Verification items for the finished model (mm, model axes). A direction names the side the tool comes from. Give positions to 0.01 mm unless a question says otherwise; leave off trailing zeros. Loops run counter-clockwise (first coordinate to the right, second up) from the corner with the lowest first, then second, coordinate; pieces in that order, holes last. Notation, with made-up numbers: (-5, 14.5) -> (17, 14.5) arc R22 cw to (17, 25.5) -> close; hole circle Ø7 at (37.5, 76). An arc over 180 degrees is marked (long way). Use one line per item in the form item = value. Start each with the question number.
from build123d import *

# Parameters (mm, degrees)
SKETCH1_R           = 5.75
SKETCH1_R_2         = 2
BOSS_EXTRUDE1_DEPTH = 10


with BuildPart() as part:
    # Sketch1 → Boss-Extrude1 (new body)
    with BuildSketch(Plane(origin=(0, 0, 0), x_dir=(1, 0, 0), z_dir=(0, 1, 0))):
        with BuildLine():
            Line((-216.382104852, 37.479356926), (33.317969978, 39.953751753))
            ThreePointArc((33.317969978, 39.953751753), (63.615239274, 9.952328714), (33.312178481, -20.043244588))
            Line((33.312178481, -20.043244588), (-216.38741399, -17.520642817))
            Line((-216.38741399, -17.520642817), (-216.382104852, 37.479356926))
        make_face()
        with Locations((33.615239414, 9.955224607)):
            Circle(SKETCH1_R, mode=Mode.SUBTRACT)
        with Locations((53.615239414, 9.955224607)):
            Circle(SKETCH1_R_2, mode=Mode.SUBTRACT)
        with Locations((43.615239414, -7.365283468)):
            Circle(SKETCH1_R_2, mode=Mode.SUBTRACT)
        with Locations((23.615239414, -7.365283468)):
            Circle(SKETCH1_R_2, mode=Mode.SUBTRACT)
        with Locations((13.615239414, 9.955224607)):
            Circle(SKETCH1_R_2, mode=Mode.SUBTRACT)
        with Locations((23.615239414, 27.275732683)):
            Circle(SKETCH1_R_2, mode=Mode.SUBTRACT)
        with Locations((43.615239414, 27.275732683)):
            Circle(SKETCH1_R_2, mode=Mode.SUBTRACT)
        with BuildLine():
            Line((-176.512574007, 22.873706291), (-121.518027204, 23.418672976))
            ThreePointArc((-121.518027204, 23.418672976), (-107.935613387, 9.968888481), (-121.52062356, -3.478273548))
            Line((-121.52062356, -3.478273548), (-176.515064128, -2.922689649))
            ThreePointArc((-176.515064128, -2.922689649), (-189.283603246, 9.976740986), (-176.512574007, 22.873706291))
        make_face(mode=Mode.SUBTRACT)
        with BuildLine():
            Line((-81.524666784, -3.882334565), (-26.530226217, -4.437918464))
            ThreePointArc((-26.530226217, -4.437918464), (-11.985090745, 9.959626398), (-26.527446362, 24.359979069))
            Line((-26.527446362, 24.359979069), (-81.521993165, 23.815012384))
            ThreePointArc((-81.521993165, 23.815012384), (-95.234126773, 9.967662409), (-81.524666784, -3.882334565))
        make_face(mode=Mode.SUBTRACT)
    extrude(amount=BOSS_EXTRUDE1_DEPTH)


solid = part.part
Item 1: Sectioned sample at D-D, the plane z = -1.5. Enter the section's corners in (x, y), and give its area (3 significant figures).
Item 2: Tool access check on faces 4 (the cylindrical face through (-107.94, 4.93, -10.27)), 5 (the flat face through (-74, 10, -30)). Record the directions out of +Z, -Z, +X, -X, +Y, -Y that give a thin tool (end or side, any length) a straight path to the whole face; none if there is none.
Item 3: Sectioned sample at C-C, the plane y = 4.5. State how many separate pieces and enclosed holes the cut face has, and give its area (3 significant figures).
Item 4: Gauge pin test, flat ends, axial feed: pin 1 Ø3 at (x, z) = (23.62, 7.37) entering from +Y; pin 2 Ø1 at (x, y) = (-99, 4) entering from +Z. Record the tip position at first contact, or that the pin passes through.
Item 5: Sectioned sample at B-B, the plane x = -130. Enter the section's corners in (y, z).
Item 6: Draft check along Z on faces 1 (the flat face through (-74, 0, -30)), 2 (the cylindrical face through (63.608, 4.93, -10.616)), 3 (the cylindrical face through (29.377, 4.93, -13.841)). Enter one of: +Z half, -Z half, draft (parallel to the pull), parting line (faces both ways), or undercut.
Item 7: Sectioned sample at A-A, the plane z = -18.5. Enter the section's corners in (x, y), and give its area (3 significant figures).
Item 8: Material ranges on line 1 (X direction, y = 3, z = -14); line 2 (X direction, y = 8.25, z = -27.5); line 3 (X direction, y = 3.5, z = -25.5), recorded low to high.
Outcome:
q1.outline = (-216.39, 0) -> (-186.11, 0) -> (-186.11, 10) -> (-216.39, 10) -> close; (-110.94, 0) -> (-92.34, 0) -> (-92.34, 10) -> (-110.94, 10) -> close; (-14.73, 0) -> (62.4, 0) -> (62.4, 10) -> (-14.73, 10) -> close
q1.area = 1,260 mm^2
q2.face_4 = +Y, -Y
q2.face_5 = +Z, -Z, +X, -X, +Y
q3.separate_pieces = 1
q3.enclosed_holes = 9
q3.area = 11,400 mm^2
q4.pin_1 = through
q4.pin_2 = 18.71
q5.outline = (0, -38.34) -> (10, -38.34) -> (10, -23.33) -> (0, -23.33) -> close; (0, 3.39) -> (10, 3.39) -> (10, 18.39) -> (0, 18.39) -> close
q6.face_1 = draft
q6.face_2 = parting line
q6.face_3 = undercut
q7.outline = (-216.38, 0) -> (-186.07, 0) -> (-186.07, 10) -> (-216.38, 10) -> close; (-110.99, 0) -> (-92.29, 0) -> (-92.29, 10) -> (-110.99, 10) -> close; (-14.79, 0) -> (62.37, 0) -> (62.37, 10) -> (-14.79, 10) -> close
q7.area = 1,260 mm^2
q8.line_1 = -216.38 to -188.64, -108.55 to -94.63, -12.56 to 29.53, 37.7 to 63.34
q8.line_2 = -216.38 to 21.63, 25.6 to 41.63, 45.6 to 57.95
q8.line_3 = -216.38 to 22.7, 24.54 to 42.7, 44.54 to 59.27
